Study the drawing (mm; zero at the part's minimum x, y, z) and answer. Coordinates: 2 decimals unless noted, no trailing zeros. Order: outer loops, then holes, each group sorted by start corner. A loop starts at its lowest first (then second) coordinate and runs counter-clockwise, first axis right, second up.
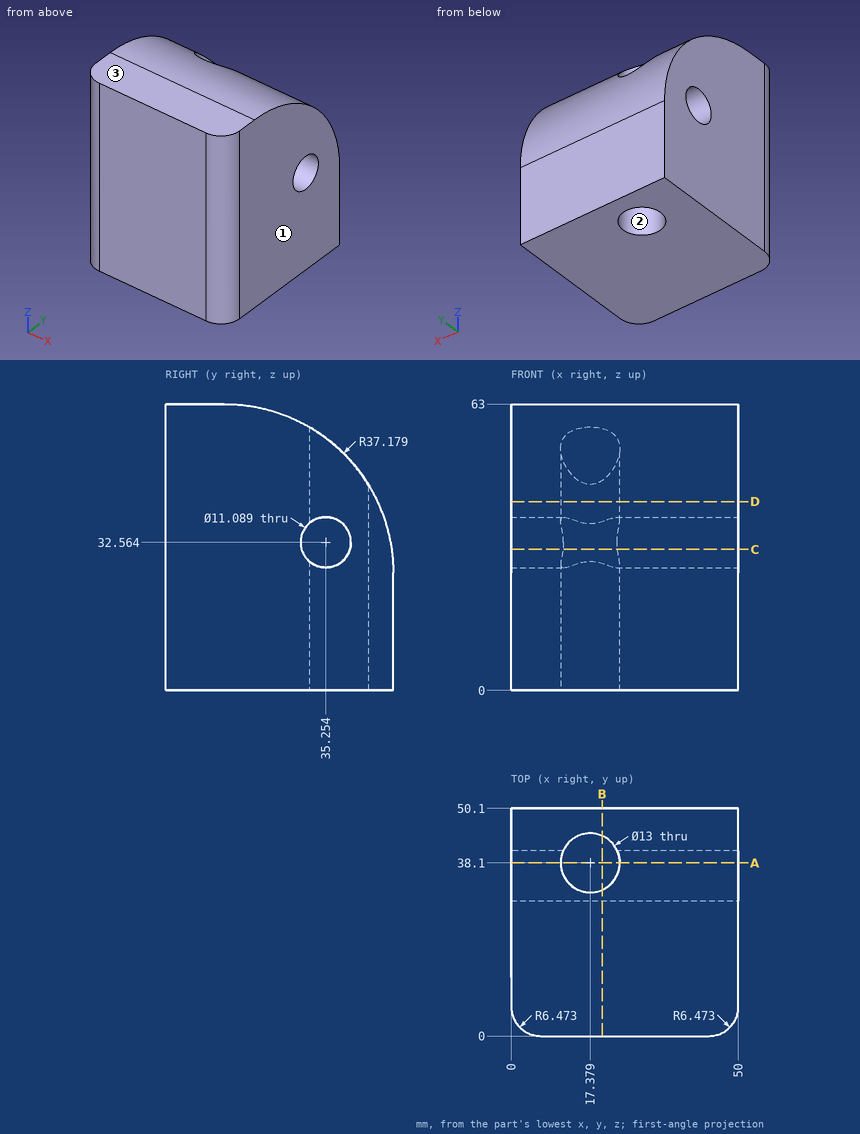
1) Flat-ended cylindrical pins translate along their axes: pin 1 Ø12 at (x, z) = (6.5, 56) entering from +Y (1 decimal); pin 2 Ø9 at (y, z) = (35.25, 32.56) entering from -X. Find the tip coordinate at first contact, or state that the pin passes through.
A:
pin 1: stops at y = 41.2
pin 2: passes through
2) A cutting plane is placed at D-D, the plane z = 41.5. Determine the outline of the cut face in (x, y), and give its area (3 significant figures).
A:
outline: (0, 6.47) arc R6.47 ccw to (6.47, 0) - (43.53, 0) arc R6.47 ccw to (50, 6.47) - (50, 46.63) - (0, 46.63) - close; hole circle Ø13 at (17.38, 38.1)
area: 2,180 mm2
3) Determine the mould class of the marked faces 1, 2 and 3 for opening direction X: pulls with the +X half, pulls with the -X half, needs draft (parallel to the pull), parting line crosses it, or undercut.
A:
face 1: pulls with the +X half
face 2: undercut
face 3: needs draft
4) A cutting plane is placed at A-A, the plane y = 38.1. Determine the outline of the cut face in (x, z).
A:
outline: (0, 0) - (10.88, 0) - (10.88, 27.81) - (0, 27.81) - close; (0, 37.32) - (10.88, 37.32) - (10.88, 53.18) - (0, 53.18) - close; (23.88, 0) - (50, 0) - (50, 27.81) - (23.88, 27.81) - close; (23.88, 37.32) - (50, 37.32) - (50, 53.18) - (23.88, 53.18) - close
5) A cutting plane is placed at C-C, the plane z = 31. Determine the outline of the cut face in (x, y) (1 decimal).
A:
outline: (0, 6.5) arc R6.5 ccw to (6.5, 0) - (43.5, 0) arc R6.5 ccw to (50, 6.5) - (50, 29.9) - (0, 29.9) - close; (0, 40.6) - (11.4, 40.6) arc R6.5 cw to (23.4, 40.6) - (50, 40.6) - (50, 49.7) - (0, 49.7) - close
6) A cutting plane is placed at B-B, the plane x = 20. Determine the outline of the cut face in (y, z) (1 decimal).
A:
outline: (0, 0) - (32.2, 0) - (32.2, 28) arc R5.5 cw to (32.2, 37.2) - (32.2, 57.6) arc R37.2 ccw to (12.9, 63) - (0, 63) - close; (44, 0) - (50.1, 0) - (50.1, 25.8) arc R37.2 ccw to (44, 46.2) - close
7) Straight lines are drawn through the part: line 1 (X direction, y = 38.1, z = 21.5); line 2 (X direction, y = 6, z = 21); line 3 (Z direction, x = 24, y = 33). For each, find the intervals that lie inside material, in ascending order.
A:
line 1: x = 0 to 10.88, 23.88 to 50
line 2: x = 0.02 to 49.98
line 3: z = 0 to 27.5, 37.63 to 57.11
